Build history of the part. All positions in model axes, mm. A direction names the side the tool comes from. Give positions to 0.01 mm unless a question says otherwise; leave off trailing zeros. Write each loop counter-clockwise with the first axis right and the second up, starting at its lowest first coordinate (ties: lowest second). Pieces come first, ordered by that corner, then holes. Notation, with made-up numbers: (53, 67) -> (106, 67) arc R23 cw to (106, 79) -> close; hole circle Ø1 at (8, 66.25). An arc over 180 degrees is marked (long way). Write item = value, one per line. Start each with the question number.
Q1. Saw through at D-D, the plane y = 25.5. List the corners of the cut face in (x, z).
Q2. Saw through at C-C, the plane z = 36. List the corners of the cut face in (x, y).
Q3. Saw through at A-A, the plane x = 95. List the corners of the cut face in (y, z), then the cut area to 3 significant figures.
Q4. Saw through at B-B, the plane x = 11. List the corners of the cut face in (y, z).
Q5. Mould opens along X. For faces 1 (the face through (88, 20, 0)), 2 (the face through (63, 20, 1)), 3 (the face through (62, 13, 0)) say: pulls with the +X half, pulls with the -X half, needs draft (parallel to the pull), parting line crosses it, or undercut.
Q6. Drop flat-ended pins along their axis: P1, Ø6, axis at x = 109.5, y = 10.5, coming from the -Z side; P2, Ø1.5, axis at x = 82, z = 16, coming from the -Y side; P3, Ø7.5, axis at x = 121, z = -3.5, coming from the -Y side. Give the stop position or say it passes through.
Q7. Wall check: line 1 (Z direction, x = 33, y = 8.5); line 2 (Y direction, x = 11, z = -28); line 3 (X direction, y = 15.75, z = 0). Give the ranges that are in metal, low to high.
Q8. Tool access for faces 4 (the face through (104.915, 28.409, -1.302)), 5 (the face through (8.615, -4.742, 36.825)), 6 (the face through (63, 5.996, -1)): list every direction of +Z, -Z, +X, -X, +Y, -Y with a clear straight run to the whole face (end or side of a thin tool).
from build123d import *

# Parameters (mm, degrees)
BOSS_EXTRUDE3_DEPTH = 40
SKETCH1_5_R         = 11
SKETCH1_5_R_2       = 6
BOSS_EXTRUDE4_DEPTH = 50
SKETCH3_W           = 31
SKETCH3_H           = 25.003683984
CUT_EXTRUDE1_DEPTH  = 62
SKETCH4_R           = 10
SKETCH4_R_2         = 7
BOSS_EXTRUDE5_DEPTH = 15
FILLET1_R           = 2
FILLET2_R           = 6
CUT_EXTRUDE2_START  = -15
SKETCH4_2_R         = 7
CUT_EXTRUDE2_DEPTH  = 15


with BuildPart() as part:
    # Sketch1 → Boss-Extrude3 (new, symmetric)
    with BuildSketch(Plane.XY):
        with BuildLine():
            Line((125, 20), (0, 20))
            Line((0, 20), (0, 5.996316016))
            ThreePointArc((0, 5.996316016), (11, 16.996316016), (22, 5.996316016))
            Line((22, 5.996316016), (103.789775753, 5.996316016))
            ThreePointArc((103.789775753, 5.996316016), (108.167652488, 4.316326302), (110, 0))
            Line((110, 0), (125, 0))
            Line((125, 0), (125, 20))
        make_face()
    extrude(amount=BOSS_EXTRUDE3_DEPTH, both=True)

    # Sketch1<5> → Boss-Extrude4 (add, symmetric)
    with BuildSketch(Plane.XY):
        with Locations((11, 5.996316016)):
            Circle(SKETCH1_5_R)
        with Locations((11, 5.996316016)):
            Circle(SKETCH1_5_R_2, mode=Mode.SUBTRACT)
    extrude(amount=BOSS_EXTRUDE4_DEPTH, both=True)

    # Sketch3 → Cut-Extrude1 (cut)
    with BuildSketch(Plane.ZY):
        with Locations((0, 7.498158008)):
            Rectangle(SKETCH3_W, SKETCH3_H)
    extrude(amount=-CUT_EXTRUDE1_DEPTH, mode=Mode.SUBTRACT)

    # Sketch4 → Boss-Extrude5 (add)
    with BuildSketch(Plane(origin=(0, 20, 0), x_dir=(1, 0, 0), z_dir=(0, 1, 0))):
        with Locations(Location((95, 0, 0), (0, 0, 270))):
            Circle(SKETCH4_R)
        with Locations(Location((95, 0, 0), (0, 0, 270))):
            Circle(SKETCH4_R_2, mode=Mode.SUBTRACT)
    extrude(amount=BOSS_EXTRUDE5_DEPTH)

    # Fillet1
    # the kernel refuses this fillet: 2 mm, written as the material it adds along each edge
    with BuildSketch(Plane(origin=(11, 5.996316016, 40), x_dir=(-1, 0, 0), z_dir=(0, -1, 0))) as fillet1_piece_1_section:
        with BuildLine():
            CenterArc((11 + FILLET1_R, -FILLET1_R), FILLET1_R, 90, 90)
            Line((11 + FILLET1_R, 0), (11, 0))
            Line((11, 0), (11, -FILLET1_R))
        make_face()
    fillet1_piece_1 = revolve(axis=Axis((11, 5.996316016, 40), (0, 0, -1)), revolution_arc=180, mode=Mode.PRIVATE)
    fillet1_piece_1 = split(fillet1_piece_1, bisect_by=Plane(origin=(0, 17.026812535, 41), z_dir=(1, 0, 0)), keep=Keep.TOP, mode=Mode.PRIVATE)
    add(fillet1_piece_1)
    with BuildSketch(Plane(origin=(95, 20, 0), x_dir=(0, 0, 1), z_dir=(-1, 0, 0))) as fillet1_piece_2:
        with BuildLine():
            CenterArc((10 + FILLET1_R, FILLET1_R), FILLET1_R, 180, 90)
            Line((10, FILLET1_R), (10, 0))
            Line((10, 0), (10 + FILLET1_R, 0))
        make_face()
    revolve(axis=Axis((95, 20, 0), (0, 1, 0)))
    with BuildSketch(Plane(origin=(11, 5.996316016, -40), x_dir=(-1, 0, 0), z_dir=(0, -1, 0))) as fillet1_piece_3_section:
        with BuildLine():
            CenterArc((11 + FILLET1_R, FILLET1_R), FILLET1_R, 180, 90)
            Line((11 + FILLET1_R, 0), (11, 0))
            Line((11, 0), (11, FILLET1_R))
        make_face()
    fillet1_piece_3 = revolve(axis=Axis((11, 5.996316016, -40), (0, 0, -1)), revolution_arc=180, mode=Mode.PRIVATE)
    fillet1_piece_3 = split(fillet1_piece_3, bisect_by=Plane(origin=(0, 17.026812535, -41), z_dir=(1, 0, 0)), keep=Keep.TOP, mode=Mode.PRIVATE)
    add(fillet1_piece_3)

    # Fillet2
    fillet2_edges = [part.edges().sort_by_distance(p)[0] for p in [
        (62, 12.998158008, -15.5),
        (62, 12.998158008, 15.5),
    ]]
    fillet(fillet2_edges, radius=FILLET2_R)

    # Sketch4<2> → Cut-Extrude2 (cut)
    with BuildSketch(Plane(origin=(0, 20, 0), x_dir=(1, 0, 0), z_dir=(0, 1, 0)).offset(CUT_EXTRUDE2_START)):
        with Locations(Location((95, 0, 0), (0, 0, 90))):
            Circle(SKETCH4_2_R)
    extrude(amount=CUT_EXTRUDE2_DEPTH, mode=Mode.SUBTRACT)


solid = part.part
Report:
q1.outline = circle Ø20 at (95, 0); hole circle Ø14 at (95, 0)
q2.outline = (0, 6) arc R11 ccw to (22, 6) -> (103.79, 6) arc R6 cw to (110, 0) -> (125, 0) -> (125, 20) -> (0, 20) -> close; hole circle Ø12 at (11, 6)
q3.outline = (6, -40) -> (20, -40) -> (20, -12) arc R2 cw to (22, -10) -> (35, -10) -> (35, -7) -> (6, -7) -> close; (6, 7) -> (35, 7) -> (35, 10) -> (22, 10) arc R2 cw to (20, 12) -> (20, 40) -> (6, 40) -> close
q3.area = 1,020 mm2
q4.outline = (-5, -50) -> (0, -50) -> (0, -15.5) -> (-5, -15.5) -> close; (-5, 15.5) -> (0, 15.5) -> (0, 50) -> (-5, 50) -> close; (12, -50) -> (17, -50) -> (17, -42) arc R2 cw to (19, -40) -> (20, -40) -> (20, -15.5) -> (12, -15.5) -> close; (12, 15.5) -> (20, 15.5) -> (20, 40) -> (19, 40) arc R2 cw to (17, 42) -> (17, 50) -> (12, 50) -> close
q5.face_1 = undercut
q5.face_2 = needs draft
q5.face_3 = pulls with the -X half
q6.P1 = -40
q6.P2 = 6
q6.P3 = 0
q7.line_1 = -40 to -15.5, 15.5 to 40
q7.line_2 = -5 to 0, 12 to 20
q7.line_3 = 62 to 88, 102 to 125
q8.face_4 = +Y
q8.face_5 = +Z
q8.face_6 = +Z, -Z, -Y
